Here's how the part is built. I have some questions about the finished solid (model axes, mm). Face numbers are marked on the shaded views. A direction names the side the tool comes from. Coordinates: 2 decimals unless noted, no trailing zeros. Order: outer loops, then holes, each group sorted by start corner. A loop starts at its lowest first (then second) coordinate and runs counter-clockwise, first axis right, second up. Notation, with made-up numbers: (-34.5, 28.5) -> (3.5, 28.5) arc R17 ccw to (3.5, 48.5) -> close; hole circle Ø5 at (38.5, 9). An arc over 180 degrees is marked (long way). One line per item, written item: value. Start each with the question number.
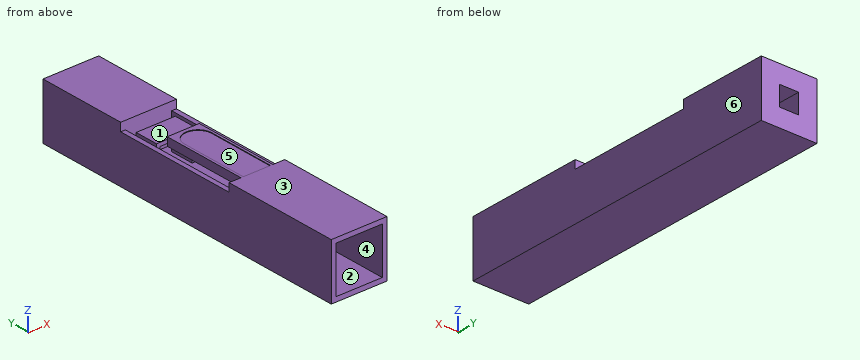
```python
from build123d import *

# Parameters (mm, degrees)
SKETCH2_W           = 2.35
SKETCH2_H           = 2.35
BOSS_EXTRUDE1_DEPTH = 7.05
PINHOLE_REACH       = 16.1
SKETCH3_W           = 0.8
SKETCH3_H           = 0.83
CUT_EXTRUDE2_DEPTH  = 0.35
SKETCH5_W           = 1.95
SKETCH5_H           = 5.3
CUT_EXTRUDE3_DEPTH  = 1.24
CUT_EXTRUDE5_DEPTH  = 0.025
SKETCH7_W           = 1.95
SKETCH7_H           = 1.95
CUT_EXTRUDE6_DEPTH  = 4
SKETCH9_W           = 0.15
SKETCH9_H           = 1
HOLDER_1_DEPTH      = 1.09
SKETCH10_W          = 1.65
SKETCH10_H          = 1
HOLDER_2_DEPTH      = 0.15


with BuildPart() as part:
    # Sketch2 → Boss-Extrude1 (new body, symmetric)
    with BuildSketch(Plane(origin=(0, 0, 0), x_dir=(1, 0, 0), z_dir=(0, 1, 0))):
        Rectangle(SKETCH2_W, SKETCH2_H)
    extrude(amount=BOSS_EXTRUDE1_DEPTH, both=True)

    # Sketch3 → Pinhole (cut, up to next)
    with BuildSketch(Plane(origin=(0, 7.05, 0), x_dir=(1, 0, 0), z_dir=(0, 1, 0)), mode=Mode.PRIVATE) as pinhole_sk1:
        Rectangle(SKETCH3_W, SKETCH3_H)
    pinhole_tool1 = extrude(pinhole_sk1.sketch, amount=-PINHOLE_REACH, mode=Mode.PRIVATE) & part.part
    add(pinhole_tool1.solids().sort_by_distance((0, 7.05, 0))[0], mode=Mode.SUBTRACT)

    # Sketch4 → Cut-Extrude2 (cut)
    with BuildSketch(Plane.XY.offset(1.175)):
        Polygon((-1.175, 3.25), (1.175, 3.25), (1.175, -2.05), (0.675, -2.05), (0.675, 1.55), (-0.675, 1.55), (-0.675, -2.05), (-1.175, -2.05), align=None)
    extrude(amount=-CUT_EXTRUDE2_DEPTH, mode=Mode.SUBTRACT)

    # Sketch5 → Cut-Extrude3 (cut)
    with BuildSketch(Plane.XY.offset(0.825)):
        with Locations((0, 0.6)):
            Rectangle(SKETCH5_W, SKETCH5_H)
    extrude(amount=-CUT_EXTRUDE3_DEPTH, mode=Mode.SUBTRACT)

    # Sketch6 → Cut-Extrude5 (cut)
    with BuildSketch(Plane.XY.offset(1.175)):
        with BuildLine():
            Line((-0.575, 0.825), (-0.575, -2.05))
            Line((-0.575, -2.05), (0.575, -2.05))
            Line((0.575, -2.05), (0.575, 0.825))
            ThreePointArc((0.575, 0.825), (0, 1.4), (-0.575, 0.825))
        make_face()
    extrude(amount=-CUT_EXTRUDE5_DEPTH, mode=Mode.SUBTRACT)

    # Sketch7 → Cut-Extrude6 (cut)
    with BuildSketch(Plane.XZ.offset(7.05)):
        Rectangle(SKETCH7_W, SKETCH7_H)
    extrude(amount=-CUT_EXTRUDE6_DEPTH, mode=Mode.SUBTRACT)

    # Sketch9 → Holder-1 (add)
    with BuildSketch(Plane.XY.offset(-0.415)):
        with Locations((-0.75, 2.4)):
            Rectangle(SKETCH9_W, SKETCH9_H)
        with Locations((0.75, 2.4)):
            Rectangle(SKETCH9_W, SKETCH9_H)
    extrude(amount=HOLDER_1_DEPTH)

    # Sketch10 → Holder-2 (add)
    with BuildSketch(Plane.XY.offset(0.675)):
        with Locations((0, 2.4)):
            Rectangle(SKETCH10_W, SKETCH10_H)
    extrude(amount=HOLDER_2_DEPTH)


solid = part.part
```
Q1. Imagine slicing it at C-C (z = -0.2). Write out the boundary of the cut face in (x, y) (3 decimals).
Q2. For P1, Ø1.1, axis at x = 0, y = 2.5, coming from the +Z side (3 decimals); P2, Ø0.6, axis at x = 0.5, y = 3, coming from the +Z side (3 decimals); P3, Ø0.6, axis at x = 0, z = -0.5, coming from the -Y side, each with a flat end and sliding along its axis, tell me the tip position at first contact or that it passes through.
Q3. I need wall thicknesses on line 1 (X direction, y = -1.75, z = 0.6) (3 decimals); line 2 (Z direction, x = -0.2, y = 1) (3 decimals); line 3 (Y direction, x = -0.5, z = 0.55). Which ranges of each line are inside material? Lowest first, please.
Q4. Imagine slicing it at B-B (x = 0). Write out the boundary of the cut face in (y, z) (3 decimals).
Q5. Imagine slicing it at D-D (y = 2.25). Write out the boundary of the cut face in (x, z) (3 decimals).
Q6. Imagine slicing it at A-A (y = -1.5). Write out the boundary of the cut face in (x, z) (3 decimals), plus the area to 3 significant figures.
Q7. If we mould it in two halves opening along Z, with no side actions, what happens to the marked faces 4, 5 and 6? For each: +Z half, -Z half, draft (parallel to the pull), parting line (faces both ways), or undercut.
Q8. For the marked faces 1, 2 and 3, which set-ups out of +Z, -Z, +X, -X, +Y, -Y let a thin tool reach every point of the face, with its end or its side?
Completed:
1. outline: (-1.175, -7.05) -> (-0.975, -7.05) -> (-0.975, -3.05) -> (-0.4, -3.05) -> (-0.4, -2.05) -> (-0.975, -2.05) -> (-0.975, 3.25) -> (-0.4, 3.25) -> (-0.4, 7.05) -> (-1.175, 7.05) -> close; (-0.825, 1.9) -> (-0.675, 1.9) -> (-0.675, 2.9) -> (-0.825, 2.9) -> close; (0.4, -3.05) -> (0.975, -3.05) -> (0.975, -7.05) -> (1.175, -7.05) -> (1.175, 7.05) -> (0.4, 7.05) -> (0.4, 3.25) -> (0.975, 3.25) -> (0.975, -2.05) -> (0.4, -2.05) -> close; (0.675, 1.9) -> (0.825, 1.9) -> (0.825, 2.9) -> (0.675, 2.9) -> close
2. P1: stops at z = 0.825
2. P2: stops at z = 1.175
2. P3: stops at y = -3.05
3. line 1: x = -1.175 to -0.975, 0.975 to 1.175
3. line 2: z = -1.175 to -0.415, 0.825 to 1.15
3. line 3: y = -3.05 to -2.05, 3.25 to 7.05
4. outline: (-7.05, -1.175) -> (7.05, -1.175) -> (7.05, -0.415) -> (-3.05, -0.415) -> (-3.05, -0.975) -> (-7.05, -0.975) -> close; (-7.05, 0.975) -> (-3.05, 0.975) -> (-3.05, 0.415) -> (-2.05, 0.415) -> (-2.05, 0.825) -> (1.55, 0.825) -> (1.55, 1.175) -> (1.4, 1.175) -> (1.4, 1.15) -> (-2.05, 1.15) -> (-2.05, 1.175) -> (-7.05, 1.175) -> close; (1.9, 0.675) -> (2.9, 0.675) -> (2.9, 0.825) -> (1.9, 0.825) -> close; (3.25, 0.415) -> (7.05, 0.415) -> (7.05, 1.175) -> (3.25, 1.175) -> close
5. outline: (-1.175, -1.175) -> (1.175, -1.175) -> (1.175, 0.825) -> (0.975, 0.825) -> (0.975, -0.415) -> (0.825, -0.415) -> (0.825, 0.825) -> (-0.825, 0.825) -> (-0.825, -0.415) -> (-0.975, -0.415) -> (-0.975, 0.825) -> (-1.175, 0.825) -> close; hole (-0.675, -0.415) -> (0.675, -0.415) -> (0.675, 0.675) -> (-0.675, 0.675) -> close
6. outline: (-1.175, -1.175) -> (1.175, -1.175) -> (1.175, 0.825) -> (0.975, 0.825) -> (0.975, -0.415) -> (-0.975, -0.415) -> (-0.975, 0.825) -> (-1.175, 0.825) -> close; (-0.675, 0.825) -> (0.675, 0.825) -> (0.675, 1.175) -> (0.575, 1.175) -> (0.575, 1.15) -> (-0.575, 1.15) -> (-0.575, 1.175) -> (-0.675, 1.175) -> close
6. area: 2.73 mm2
7. face 4: undercut
7. face 5: +Z half
7. face 6: draft
8. face 1: +Z, +X, -X
8. face 2: -Y
8. face 3: +Z, +X, -X, +Y, -Y
